```python
from build123d import *

# Parameters (mm, degrees)
BOSS_EXTRUDE1_DEPTH = 4
SKETCH2_R           = 256
CUT_EXTRUDE1_DEPTH  = 50
EXTRUDE_THIN1_START = -10
SKETCH3_R           = 258
SKETCH3_R_2         = 256
EXTRUDE_THIN1_DEPTH = 10
SKETCH4_R           = 4.5
BOSS_EXTRUDE2_DEPTH = 30
CIRPATTERN1_COUNT   = 12


with BuildPart() as part:
    # Sketch1 → Boss-Extrude1 (new body)
    with BuildSketch(Plane.XY):
        with BuildLine():
            Line((865.269127642, 521.057153497), (865.269127642, 757.057153497))
            ThreePointArc((865.269127642, 757.057153497), (782.812941082, 1010.7278743), (545.269127642, 1132.057153497))
            ThreePointArc((545.269127642, 1132.057153497), (233.519744905, 1040.749713195), (75.269127642, 757.057153497))
            ThreePointArc((75.269127642, 757.057153497), (198.687627947, 391.283260157), (545.269127642, 221.271697797))
            ThreePointArc((545.269127642, 221.271697797), (725.219790584, 211.189307063), (905.269127642, 203.057153497))
            Line((905.269127642, 203.057153497), (905.269127642, 521.057153497))
            Line((905.269127642, 521.057153497), (865.269127642, 521.057153497))
        make_face()
    extrude(amount=BOSS_EXTRUDE1_DEPTH)

    # Sketch2 → Cut-Extrude1 (cut)
    with BuildSketch(Plane.XY.offset(4)):
        with Locations((545.269127642, 758.057153497)):
            Circle(SKETCH2_R)
    extrude(amount=-CUT_EXTRUDE1_DEPTH, mode=Mode.SUBTRACT)

    # Sketch3 → Extrude-Thin1 (add)
    with BuildSketch(Plane(origin=(0, 0, 0), x_dir=(-1, 0, 0), z_dir=(0, 0, -1)).offset(EXTRUDE_THIN1_START)):
        with Locations((-545.269127642, 758.057153497)):
            Circle(SKETCH3_R)
        with Locations((-545.269127642, 758.057153497)):
            Circle(SKETCH3_R_2, mode=Mode.SUBTRACT)
    extrude(amount=EXTRUDE_THIN1_DEPTH)

    # Sketch4 → Boss-Extrude2 (add)
    with BuildSketch(Plane(origin=(0, 0, 0), x_dir=(-1, 0, 0), z_dir=(0, 0, -1))):
        with Locations((-545.269127642, 1033.057153497)):
            Circle(SKETCH4_R)
    boss_extrude2 = extrude(amount=BOSS_EXTRUDE2_DEPTH)

    # CirPattern1: Boss-Extrude2 ×12 about axis
    cirpattern1_axis = Axis((545.269127642, 758.057153497, 0), (0, 0, 1))
    for i in range(1, CIRPATTERN1_COUNT):
        add(boss_extrude2.rotate(cirpattern1_axis, i * 360 / CIRPATTERN1_COUNT))


solid = part.part
```
Read the model definition and answer for the solid it produces. Units are mm, in the model's axes. Give positions to 0.01 mm unless a question says otherwise; leave off trailing zeros. Order: outer loops, then holes, each group sorted by start corner. A loop starts at its lowest first (then second) coordinate and runs counter-clockwise, first axis right, second up. Notation, with made-up numbers: (23.5, -30.75) -> (44.5, -30.75) arc R11 cw to (44.5, -12.75) -> close; hole circle Ø11 at (23.5, 46.5). An arc over 180 degrees is marked (long way). One line per item, written item: value. Start each with the question number.
(1) The part is cut by section B-B (x = 369). Determine the outline of the cut face in (y, z), and give its area (3 significant figures).
(2) Flat-ended cylindrical pins translate along their axes: P1, Ø2, axis at x = 891, z = 1.5, coming from the +Y side; P2, Ø4.5, axis at y = 647, z = 2, coming from the +X side; P3, Ø8, axis at x = 721.5, z = -1.5, coming from the -Y side; P4, Ø8, axis at y = 969, z = -6.5, coming from the +X side. Find the tip coordinate at first contact, or state that the pin passes through.
(3) Straight lines are drawn through the part: L1, parallel to X at y = 758, z = -7.5; L2, parallel to Z at x = 472, y = 364.5; L3, parallel to X at y = 858, z = 6.5. For each, find the intervals that lie inside material, in ascending order.
(4) The part is cut by section A-A (z = -7.5). State how many separate pieces and enclosed holes the cut face has, and give its area (3 significant figures).
(5) The part is cut by section D-D (x = 192). Determine the outline of the cut face in (y, z).
(6) The part is cut by section C-C (y = 592). Determine the outline of the cut face in (x, z), and give its area (3 significant figures).
Taken from the geometry:
1. outline: (265.02, 0) -> (572.41, 0) -> (572.41, 10) -> (569.66, 10) -> (569.66, 4) -> (265.02, 4) -> close; (943.71, 0) -> (1113.55, 0) -> (1113.55, 4) -> (946.45, 4) -> (946.45, 10) -> (943.71, 10) -> close
1. area: 1,940 mm^2
2. P1: y = 521.06
2. P2: x = 865.27
2. P3: y = 211.19
2. P4: through
3. L1: 265.77 to 274.77, 815.77 to 824.77
3. L2: 0 to 4
3. L3: 307.41 to 309.58, 780.95 to 783.13
4. separate pieces: 12
4. enclosed holes: 0
4. area: 763 mm^2
5. outline: (399.07, 0) -> (1002.91, 0) -> (1002.91, 4) -> (399.07, 4) -> close
6. outline: (91.28, 0) -> (350.43, 0) -> (350.43, 10) -> (347.81, 10) -> (347.81, 4) -> (91.28, 4) -> close; (740.11, 0) -> (865.27, 0) -> (865.27, 4) -> (742.73, 4) -> (742.73, 10) -> (740.11, 10) -> close
6. area: 1,570 mm^2
